Check sheet for the modelled part. Datum: model origin and axes. Units: mm. Round coordinates to 2 decimals unless told otherwise and drop trailing zeros. Loops run counter-clockwise (first coordinate to the right, second up) from the corner with the lowest first, then second, coordinate; pieces in that order, holes last. Notation, with made-up numbers: (6, -12.75) -> (13, -12.75) arc R15 ccw to (13, 14.25) -> close; hole circle Ø6 at (-4, 27.5). An arc over 180 degrees is marked (long way). Use one line per item in the form item = value. Start each with the question number.
(1) Sectioned sample at A-A (z = -390). Record the cut outline in (x, y).
(2) Material ranges on probe 1 along X at (y, z) = (3, -390); probe 2 along Z at (x, y) = (-994, 3.15); probe 3 along Z at (x, y) = (994, 1.55), recorded low to high. Write a range as [from, to].
(3) Sectioned sample at D-D (z = 262.5). Record the cut outline in (x, y), and give its area (3 significant figures).
(4) Sectioned sample at C-C (x = -994). Record the cut outline in (y, z).
(5) Sectioned sample at B-B (x = 994). Record the cut outline in (y, z).
Autodesk Inventor part; units mm, degrees
ref_plane "YZ Plane" through (0, 0, 0) normal (1, 0, 0) x (0, 1, 0)
ref_plane "XZ Plane" through (0, 0, 0) normal (0, 1, 0) x (-1, 0, 0)
ref_plane "XY Plane" through (0, 0, 0) normal (0, 0, 1) x (1, 0, 0)
sketch "Sketch1" plane through (0, 0, 0) normal (0, 1, 0) x (-1, 0, 0)
  line L0 (1244, -740) -> (-1244, -740)
  line L1 (-1244, -740) -> (-1244, 740)
  line L2 (-1244, 740) -> (1244, 740)
  line L3 (1244, 740) -> (1244, -740)
  line L4 (1244, -740) -> (-1244, 740) construction
  line L5 (-1244, -740) -> (1244, 740) construction
  point P0 (0, 0)
  dimension "d0" = 2488
  dimension "d1" = 1480
extrude "Plate1" add sketch "Sketch1" along normal blind 4
sketch "Sketch2" plane through (0, 4, 0) normal (0, 1, 0) x (1, 0, 0)
  line L0 (-1244, -740) -> (-1244, 740) construction
  line L1 (1244, -740) -> (-1244, -740) construction
  line L2 (1244, 740) -> (1244, -740) construction
  line L3 (-1244, 740) -> (1244, 740) construction
  circle A0 centre (-994, 390) radius 160
  point P0 (0, 0)
  dimension "d6" = 320
  dimension "d7" = 250
  dimension "d8" = 350
extrude "Cut1" cut sketch "Sketch2" against normal blind 4
mirror "Mirror1" about plane through (0, 0, 0) normal (1, 0, 0) of "Cut1"
mirror "Mirror2" about plane through (0, 0, 0) normal (0, 0, 1) of "Cut1"
fillet "Corner Round1" radius 20 4 edges at (-1244, 2, 740) (-1244, 2, -740) (1244, 2, -740) (1244, 2, 740)
equation "\"d9\" = Thickness"
equation "\"d2\" = Thickness"
equation "\"BendRadius\" = Thickness"
equation "\"BendReliefWidth\" = Thickness"
equation "\"BendReliefDepth\" = 0.5 * Thickness"
equation "\"CornerReliefSize\" = 4 * Thickness"
equation "\"MinimumRemnant\" = 2 * Thickness"
equation "\"TransitionRadius\" = BendRadius"
equation "\"JacobiRadiusSize\" = BendRadius"
equation "\"GapSize\" = Thickness"
properties part number "GBK-RK-0021 bottom"
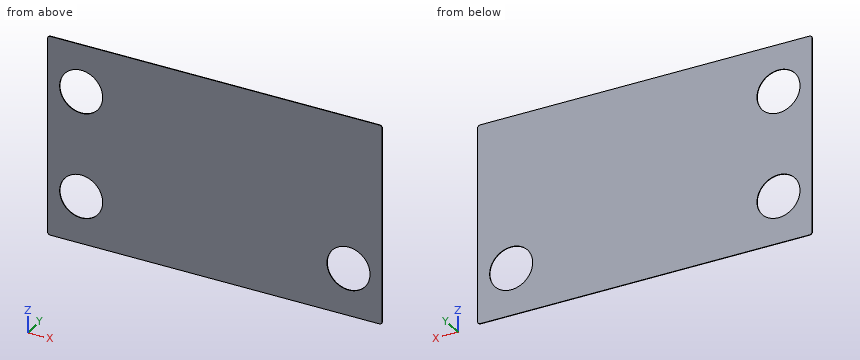
Checks:
q1.outline = (-1244, 0) -> (-1154, 0) -> (-1154, 4) -> (-1244, 4) -> close; (-834, 0) -> (834, 0) -> (834, 4) -> (-834, 4) -> close; (1154, 0) -> (1244, 0) -> (1244, 4) -> (1154, 4) -> close
q2.probe_1 = [-1244, -1154], [-834, 834], [1154, 1244]
q2.probe_2 = [-740, -550], [-230, 230], [550, 740]
q2.probe_3 = [-740, -550], [-230, 740]
q3.outline = (-1244, 0) -> (-1090.66, 0) -> (-1090.66, 4) -> (-1244, 4) -> close; (-897.34, 0) -> (1244, 0) -> (1244, 4) -> (-897.34, 4) -> close
q3.area = 9,180 mm2
q4.outline = (0, -740) -> (4, -740) -> (4, -550) -> (0, -550) -> close; (0, -230) -> (4, -230) -> (4, 230) -> (0, 230) -> close; (0, 550) -> (4, 550) -> (4, 740) -> (0, 740) -> close
q5.outline = (0, -740) -> (4, -740) -> (4, -550) -> (0, -550) -> close; (0, -230) -> (4, -230) -> (4, 740) -> (0, 740) -> close
